from build123d import *

# Parameters (mm, degrees)
F1_DEPTH = 16.29


with BuildPart() as f1:
    # F0 (on Front) → F1 (new body, symmetric)
    with BuildSketch(Plane.XZ):
        with BuildLine():
            Line((-29.761402, -6.935), (35.475, -6.935))
            Line((35.475, -6.935), (35.475, 6.935))
            Line((35.475, 6.935), (-29.761402, 6.935))
            ThreePointArc((-29.761402, 6.935), (-33.862627, 4.492756), (-35.475, 0))
            ThreePointArc((-35.475, 0), (-33.862627, -4.492756), (-29.761402, -6.935))
        make_face()
    extrude(amount=F1_DEPTH, both=True)


solid = f1.part
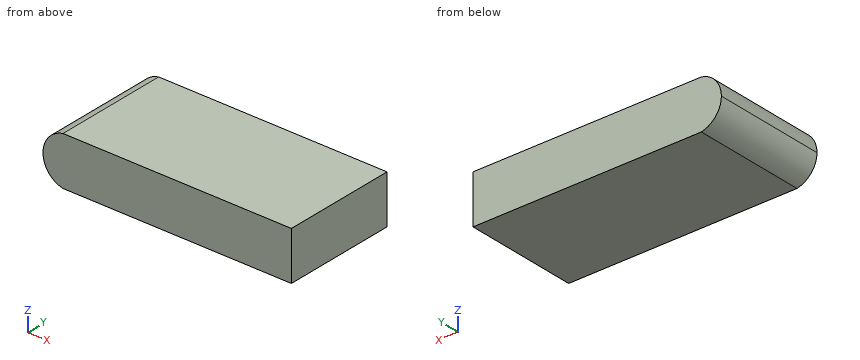
Here's how the part is built. I have some questions about the finished solid (model axes, mm). Coordinates: 2 decimals unless noted, no trailing zeros. Order: outer loops, then holes, each group sorted by start corner. A loop starts at its lowest first (then second) coordinate and runs counter-clockwise, first axis right, second up. Notation, with made-up numbers: M 38.25,65.5 L 42.25,65.5 A13 ccw 42.25,72.5 Z; hole C 24.5,-12.75 d2. An arc over 180 degrees is marked long. Answer as CSV lines item,"result".
Item 1: Imagine slicing it at A-A on y = -6. Write out the boundary of the cut face in (x, z) (3 decimals), plus the area to 3 significant figures.
Results found:
outline,"M -29.761,-6.935 L 35.475,-6.935 L 35.475,6.935 L -29.761,6.935 A7.066 ccw Z"
area,"964 mm2"
Item 2: If I drill on line 1 (X direction, y = -15, z = 3.75) (3 decimals); line 2 (X direction, y = -13.5, z = -3.25) (3 decimals), over which ranges is the centre line in solid material (lowest first)?
Results found:
line 1,"-34.398 to 35.475"
line 2,"-34.683 to 35.475"
Item 3: Imagine slicing it at B-B on z = -4. Write out the boundary of the cut face in (x, y) (3 decimals), plus the area to 3 significant figures.
Results found:
outline,"M -34.234,-16.29 L 35.475,-16.29 L 35.475,16.29 L -34.234,16.29 Z"
area,"2,270 mm2"
